The drawing under review shows one solid part. Ordinate dimensions are in mm from its lowest x, y, z. Coordinates: 2 decimals unless noted, no trailing zeros. Write each loop counter-clockwise with the first axis right and the second up, starting at its lowest first coordinate (ties: lowest second). Pieces come first, ordered by that corner, then holes. Notation, with made-up numbers: (28.25, 48) - (36.25, 48) arc R27 cw to (36.25, 70) - close; hole circle Ø7 at (-25, 44). An arc over 180 degrees is marked (long way). Put each result on its own line as item: value. Start each with the question number.
Item 1: Consider section B-B on y = 508. Give the boundary of the cut face in (x, z).
Item 2: To check wall thickness, follow L1, parallel to X at y = 507.5, z = 19.5; L2, parallel to X at y = 837, z = 24; L3, parallel to Y at x = 305, z = 31.5. State the ranges of each line that lie inside material, in increasing order. Write a range as [from, to].
Item 3: For pin 1 (8 mm diameter, centred on x = 256, z = 20.5, fed in from +Y); pin 2 (1.5 mm diameter, centred on x = 304, z = 20.5, fed in from +Y); pin 3 (11.5 mm diameter, centred on x = 191, z = 10, fed in from +Y), all flat-tipped, find the tip position at first contact; note any pin that passes through.
Item 4: Consider section A-A on z = 10.5. Give the boundary of the cut face in (x, y), then the cut area to 3 significant figures.
Item 5: Consider section D-D on x = 172. Give the boundary of the cut face in (y, z), then the cut area to 3 significant figures.
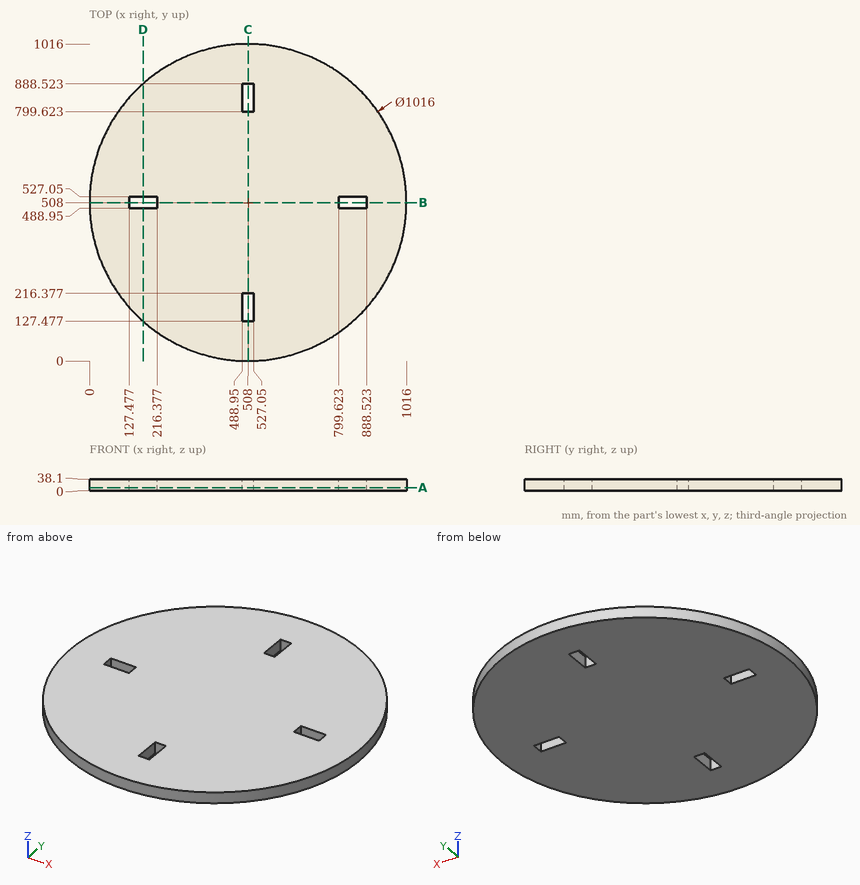
Report:
1. outline: (0, 0) - (127.48, 0) - (127.48, 38.1) - (0, 38.1) - close; (216.38, 0) - (799.62, 0) - (799.62, 38.1) - (216.38, 38.1) - close; (888.52, 0) - (1016, 0) - (1016, 38.1) - (888.52, 38.1) - close
2. L1: [0, 127.48], [216.38, 799.62], [888.52, 1016]
2. L2: [120.93, 488.95], [527.05, 895.07]
2. L3: [42.32, 973.68]
3. pin 1: y = 951.35
3. pin 2: y = 973.57
3. pin 3: y = 909.48
4. outline: circle Ø1016 at (508, 508); hole (127.48, 488.95) - (216.38, 488.95) - (216.38, 527.05) - (127.48, 527.05) - close; hole (488.95, 127.48) - (527.05, 127.48) - (527.05, 216.38) - (488.95, 216.38) - close; hole (488.95, 799.62) - (527.05, 799.62) - (527.05, 888.52) - (488.95, 888.52) - close; hole (799.62, 488.95) - (888.52, 488.95) - (888.52, 527.05) - (799.62, 527.05) - close
4. area: 797,000 mm²
5. outline: (126.99, 0) - (488.95, 0) - (488.95, 38.1) - (126.99, 38.1) - close; (527.05, 0) - (889.01, 0) - (889.01, 38.1) - (527.05, 38.1) - close
5. area: 27,600 mm²
